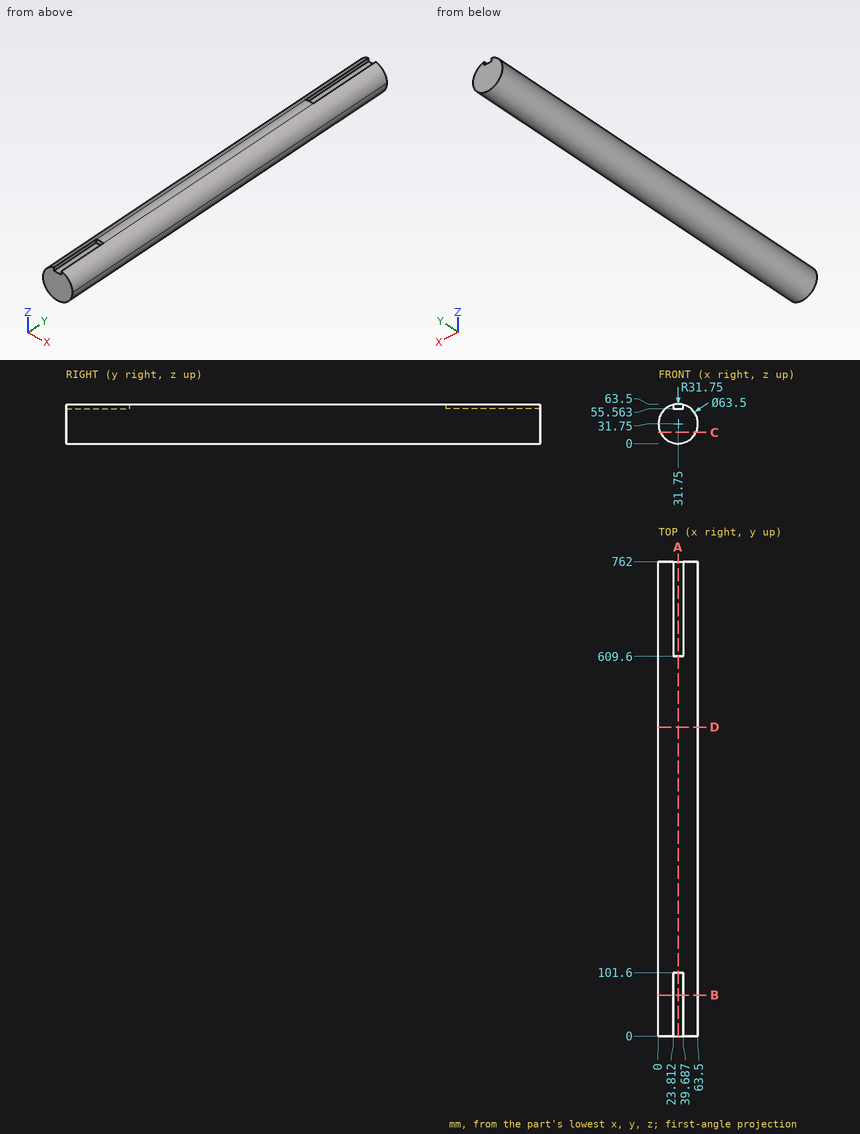
Here's the drawing with two shaded views (mm, measured from the low corner). I have some questions. Round coordinates to 2 decimals unless told otherwise and drop trailing zeros. Loops run counter-clockwise (first coordinate to the right, second up) from the corner with the lowest first, then second, coordinate; pieces in that order, holes last. Notation, with made-up numbers: M 42,38.5 L 49,38.5 A3 ccw 49,42.5 Z; hole C -35,-14 d10. An arc over 180 degrees is marked long. Put each result on its own line as item: value.
Q1. Imagine slicing it at B-B (y = 65.5). Write out the boundary of the cut face in (x, z).
Check result:
outline: M 23.81,55.56 L 23.81,62.49 A31.75 ccw long 63.5,31.75 A31.75 ccw 39.69,62.49 L 39.69,55.56 Z
Q2. Imagine slicing it at D-D (y = 496). Write out the boundary of the cut face in (x, z), then the cut area to 3 significant figures.
Check result:
outline: M 23.81,62.49 A31.75 ccw long 63.5,31.75 A31.75 ccw 39.69,62.49 A31.75 ccw Z
area: 3,170 mm2
Q3. Imagine slicing it at A-A (x = 31.75). Write out the boundary of the cut face in (y, z).
Check result:
outline: M 0,0 L 762,0 L 762,55.56 L 609.6,55.56 L 609.6,63.5 L 101.6,63.5 L 101.6,55.56 L 0,55.56 Z
Q4. I need wall thicknesses on probe 1 along X at (y, z) = (682, 34); probe 2 along X at (y, z) = (722, 57) (1 decimal); probe 3 along X at (y, z) = (217, 32.5). Which ranges of each line are inside material? Lowest first, please.
Check result:
probe 1: 0.08 to 63.42
probe 2: 12.5 to 23.8, 39.7 to 51
probe 3: 0.01 to 63.49
Q5. For pin 1 (4 mm diameter, centred on x = 35.5, z = 61, fed in from +Y); pin 2 (3 mm diameter, centred on y = 89, z = 49, fed in from +X); pin 3 (8 mm diameter, centred on x = 55, y = 206.5, fed in from +Z); pin 4 (4 mm diameter, centred on x = 29, z = 57.5, fed in from -Y), each with a flat end and sliding along its axis, tell me the tip position at first contact or that it passes through.
Check result:
pin 1: y = 609.6
pin 2: x = 59.32
pin 3: z = 57
pin 4: y = 0
Q6. Imagine slicing it at C-C (z = 18). Write out the boundary of the cut face in (x, y).
Check result:
outline: M 3.13,0 L 60.37,0 L 60.37,762 L 3.13,762 Z
